```python
from build123d import *

# Parameters (mm, degrees)
SKETCH1_W           = 36.5
SKETCH1_H           = 18
BOSS_EXTRUDE1_DEPTH = 5
SKETCH2_W           = 32.5
SKETCH2_H           = 14
CUT_EXTRUDE1_DEPTH  = 2.4
SKETCH3_W           = 5
SKETCH3_H           = 3
BOSS_EXTRUDE2_DEPTH = 2.4
CUT_EXTRUDE2_REACH  = 4
SKETCH4_W           = 5.5
SKETCH4_H           = 5
SKETCH5_W           = 3.6
SKETCH5_H           = 5
SKETCH5_W_2         = 4.8
SKETCH5_H_2         = 6
CUT_EXTRUDE3_DEPTH  = 1.6
SKETCH6_W           = 14.6
SKETCH6_H           = 5
SKETCH6_W_2         = 4.4
BOSS_EXTRUDE3_DEPTH = 4
SKETCH7_W           = 10
SKETCH7_H           = 5
BOSS_EXTRUDE4_DEPTH = 4


with BuildPart() as part:
    # Sketch1 → Boss-Extrude1 (new body)
    with BuildSketch(Plane(origin=(0, 0, 0), x_dir=(1, 0, 0), z_dir=(0, 1, 0))):
        with Locations((18.25, 9)):
            Rectangle(SKETCH1_W, SKETCH1_H)
    extrude(amount=-BOSS_EXTRUDE1_DEPTH)

    # Sketch2 → Cut-Extrude1 (cut)
    with BuildSketch(Plane(origin=(0, 0, 0), x_dir=(1, 0, 0), z_dir=(0, 1, 0))):
        with Locations((18.25, 9)):
            Rectangle(SKETCH2_W, SKETCH2_H)
    extrude(amount=-CUT_EXTRUDE1_DEPTH, mode=Mode.SUBTRACT)

    # Sketch3 → Boss-Extrude2 (add)
    with BuildSketch(Plane(origin=(0, -2.4, 0), x_dir=(1, 0, 0), z_dir=(0, 1, 0))):
        with Locations((10.5, 6)):
            Rectangle(SKETCH3_W, SKETCH3_H)
    extrude(amount=BOSS_EXTRUDE2_DEPTH)

    # Sketch4 → Cut-Extrude2 (cut, up to next)
    with BuildSketch(Plane(origin=(0, 0, -2), x_dir=(-1, 0, 0), z_dir=(0, 0, -1)), mode=Mode.PRIVATE) as cut_extrude2_sk1:
        with Locations((-23.35, -2.5)):
            Rectangle(SKETCH4_W, SKETCH4_H)
    cut_extrude2_tool1 = extrude(cut_extrude2_sk1.sketch, amount=-CUT_EXTRUDE2_REACH, mode=Mode.PRIVATE) & part.part
    add(cut_extrude2_tool1.solids().sort_by_distance((23.35, -2.5, -2))[0], mode=Mode.SUBTRACT)

    # Sketch5 → Cut-Extrude3 (cut)
    with BuildSketch(Plane(origin=(0, -2.4, 0), x_dir=(1, 0, 0), z_dir=(0, 1, 0))):
        with Locations((3.8, 4.5)):
            Rectangle(SKETCH5_W, SKETCH5_H)
        with Locations((32.1, 5)):
            Rectangle(SKETCH5_W_2, SKETCH5_H_2)
    extrude(amount=-CUT_EXTRUDE3_DEPTH, mode=Mode.SUBTRACT)

    # Sketch6 → Boss-Extrude3 (add)
    with BuildSketch(Plane.XY):
        with Locations((10.3, -2.5)):
            Rectangle(SKETCH6_W, SKETCH6_H)
        with Locations((31.3, -2.5)):
            Rectangle(SKETCH6_W_2, SKETCH6_H)
    extrude(amount=BOSS_EXTRUDE3_DEPTH)

    # Sketch7 → Boss-Extrude4 (add)
    with BuildSketch(Plane(origin=(36.5, 0, 0), x_dir=(0, 0, -1), z_dir=(1, 0, 0))):
        with Locations((9, -2.5)):
            Rectangle(SKETCH7_W, SKETCH7_H)
    extrude(amount=BOSS_EXTRUDE4_DEPTH)


solid = part.part
```
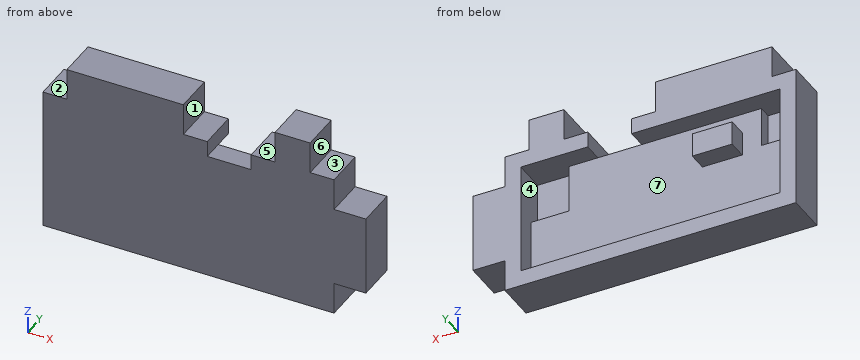
Here's how the part is built. I have some questions about the finished solid (model axes, mm). Face numbers are marked on the shaded views. A direction names the side the tool comes from. Round coordinates to 2 decimals unless told otherwise and drop trailing zeros. Loops run counter-clockwise (first coordinate to the right, second up) from the corner with the lowest first, then second, coordinate; pieces in that order, holes last.
1. Suppose I cut it at A-A, the plane y = -2.85. Please give me the cut outline in (x, z).
Answers:
outline: (0, -18) - (36.5, -18) - (36.5, -14) - (40.5, -14) - (40.5, -4) - (36.5, -4) - (36.5, 0) - (33.5, 0) - (33.5, 4) - (29.1, 4) - (29.1, 0) - (26.1, 0) - (26.1, -2) - (20.6, -2) - (20.6, 0) - (17.6, 0) - (17.6, 4) - (3, 4) - (3, 0) - (0, 0) - close; hole (2, -7) - (5.6, -7) - (5.6, -2) - (2, -2) - close; hole (29.7, -8) - (34.5, -8) - (34.5, -2) - (29.7, -2) - close
2. Will these pins go through, and if not, where does the flat tip stop? pin 1 (1 mm diameter, centred on y = -2, z = -1, fed in from +X); pin 2 (2.5 mm diameter, centred on x = 19, y = -3, fed in from +Z); pin 3 (2 mm diameter, centred on x = 38.5, y = -1.5, fed in from -Z).
Answers:
pin 1: stops at x = 36.5
pin 2: stops at z = 0
pin 3: stops at z = -14
3. If I drill on probe 1 along Z at (x, y) = (11, -1.8); probe 2 along X at (y, z) = (-3.45, -6.75); probe 3 along X at (y, z) = (-3.1, -2.5), over which ranges is the centre line in solid material (lowest first)?
Answers:
probe 1: z = -18 to -16, -7.5 to -4.5, -2 to 4
probe 2: x = 0 to 2, 5.6 to 29.7, 34.5 to 40.5
probe 3: x = 0 to 2, 5.6 to 29.7, 34.5 to 36.5
4. Suppose I cut it at D-D, the plane z = -9. Please give me the cut outline in (x, y), and give its area (4 significant figures).
Answers:
outline: (0, -5) - (40.5, -5) - (40.5, 0) - (34.5, 0) - (34.5, -2.4) - (2, -2.4) - (2, 0) - (0, 0) - close
area: 124.5 mm2
5. Suppose I cut it at B-B, the plane z = 1.25. Please give me the cut outline in (x, y).
Answers:
outline: (3, -5) - (17.6, -5) - (17.6, 0) - (3, 0) - close; (29.1, -5) - (33.5, -5) - (33.5, 0) - (29.1, 0) - close
6. Thinking about a two-plate mould opening in Z: for the marked faces 4, 5, 6 and 7, which applies, released by +Z, released by -Z, zero draft, split by the parting line, or undercut?
Answers:
face 4: undercut
face 5: released by +Z
face 6: zero draft
face 7: undercut
7. For the marked faces 1, 2 and 3, which set-ups out of +Z, -Z, +X, -X, +Y, -Y let a thin tool reach every point of the face, with its end or its side?
Answers:
face 1: +Z, +Y, -Y
face 2: +Z, -X, +Y, -Y
face 3: +Z, +X, +Y, -Y
8. Suppose I cut it at C-C, the plane x = 18. Please give me the cut outline in (y, z), and give its area (3 significant figures).
Answers:
outline: (-5, -18) - (0, -18) - (0, -16) - (-2.4, -16) - (-2.4, -2) - (0, -2) - (0, 0) - (-5, 0) - close
area: 56.4 mm2
